from build123d import *

# Parameters (mm, degrees)
BOSS_EXTRUDE1_START = 5
BOSS_EXTRUDE1_DEPTH = 1
SKETCH1_4_W         = 1
SKETCH1_4_H         = 4.3053
BOSS_EXTRUDE2_DEPTH = 5
BOSS_EXTRUDE3_DEPTH = 1.5875


with BuildPart() as part:
    # Sketch1 → Boss-Extrude1 (new body)
    with BuildSketch(Plane(origin=(0, 0, 0), x_dir=(1, 0, 0), z_dir=(0, 1, 0)).offset(BOSS_EXTRUDE1_START)):
        Polygon((13.035, -4), (13.035, 4), (18.035, 4), (18.035, 13.796348116), (3.75, 13.796348116), (3.75, -13.796348116), (18.035, -13.796348116), (18.035, -4), align=None)
    extrude(amount=BOSS_EXTRUDE1_DEPTH)

    # Sketch1<4> → Boss-Extrude2 (add)
    with BuildSketch(Plane(origin=(0, 0, 0), x_dir=(1, 0, 0), z_dir=(0, 1, 0))):
        with Locations((4.25, 0)):
            Rectangle(SKETCH1_4_W, SKETCH1_4_H)
        Polygon((3.75, 3.15265), (3.75, 2.15265), (4.75, 2.15265), (4.75, 12.796348116), (17.035, 12.796348116), (18.035, 12.796348116), (18.035, 13.796348116), (3.75, 13.796348116), align=None)
        Polygon((4.75, -2.15265), (3.75, -2.15265), (3.75, -3.15265), (3.75, -13.796348116), (18.035, -13.796348116), (18.035, -12.796348116), (17.035, -12.796348116), (4.75, -12.796348116), align=None)
    extrude(amount=BOSS_EXTRUDE2_DEPTH)

    # Sketch1<5> → Boss-Extrude3 (add)
    with BuildSketch(Plane(origin=(0, 0, 0), x_dir=(1, 0, 0), z_dir=(0, 1, 0))):
        with BuildLine():
            Line((2.303323685, 2.15265), (3.75, 2.15265))
            Line((3.75, 2.15265), (3.75, 3.15265))
            Line((3.75, 3.15265), (0, 3.15265))
            ThreePointArc((0, 3.15265), (1.255517821, 2.891863936), (2.303323685, 2.15265))
        make_face()
        with BuildLine():
            Line((3.75, -2.15265), (3.75, 2.15265))
            Line((3.75, 2.15265), (2.303323685, 2.15265))
            ThreePointArc((2.303323685, 2.15265), (2.932641765, 1.157071434), (3.15265, 0))
            ThreePointArc((3.15265, 0), (2.932641765, -1.157071434), (2.303323685, -2.15265))
            Line((2.303323685, -2.15265), (3.75, -2.15265))
        make_face()
        with BuildLine():
            Line((3.75, -3.15265), (3.75, -2.15265))
            Line((3.75, -2.15265), (2.303323685, -2.15265))
            ThreePointArc((2.303323685, -2.15265), (1.255517821, -2.891863936), (0, -3.15265))
            Line((0, -3.15265), (3.75, -3.15265))
        make_face()
        with BuildLine():
            ThreePointArc((3.15265, 0), (2.932641765, 1.157071434), (2.303323685, 2.15265))
            Line((2.303323685, 2.15265), (0, 2.15265))
            ThreePointArc((0, 2.15265), (1.522153413, 1.522153413), (2.15265, 0))
            ThreePointArc((2.15265, 0), (1.522153413, -1.522153413), (0, -2.15265))
            Line((0, -2.15265), (2.303323685, -2.15265))
            ThreePointArc((2.303323685, -2.15265), (2.932641765, -1.157071434), (3.15265, 0))
        make_face()
        with BuildLine():
            ThreePointArc((0, -2.15265), (-2.15265, 0), (0, 2.15265))
            Line((0, 2.15265), (0, 3.15265))
            ThreePointArc((0, 3.15265), (-3.15265, 0), (0, -3.15265))
            Line((0, -3.15265), (0, -2.15265))
        make_face()
        with BuildLine():
            Line((0, 2.15265), (2.303323685, 2.15265))
            ThreePointArc((2.303323685, 2.15265), (1.255517821, 2.891863936), (0, 3.15265))
            Line((0, 3.15265), (0, 2.15265))
        make_face()
        with BuildLine():
            ThreePointArc((0, -3.15265), (1.255517821, -2.891863936), (2.303323685, -2.15265))
            Line((2.303323685, -2.15265), (0, -2.15265))
            Line((0, -2.15265), (0, -3.15265))
        make_face()
    extrude(amount=BOSS_EXTRUDE3_DEPTH)


solid = part.part
Can you work these out from the model? Positions are in its coordinate system, mm. A direction names the side the tool comes from. Give positions to 0.01 mm unless a question says otherwise; leave off trailing zeros. Loops run counter-clockwise (first coordinate to the right, second up) from the corner with the lowest first, then second, coordinate; pieces in that order, holes last. Notation, with made-up numbers: (-16, -36.5) - (2, -36.5) arc R23 ccw to (2, -4.5) - close; hole circle Ø11 at (30, -18). An arc over 180 degrees is marked (long way). Answer as a JSON object with one key per item and string values.
Q1. If I drill on L1, parallel to Z at x = 16.5, y = 4.45; L2, parallel to X at y = 3.6, z = -11; L3, parallel to X at y = 5.55, z = 10 (3 decimals), over which ranges is the centre line in solid material (lowest first)?
Geometry says:
{"L1": "-13.8 to -12.8, 12.8 to 13.8", "L2": "3.75 to 4.75", "L3": "3.75 to 18.035"}
Q2. Will these pins go through, and if not, where does the flat tip stop? P1, Ø1.7, axis at x = 2, y = 0.5, coming from the -Z side; P2, Ø10.5, axis at x = 13.5, z = -4.5, coming from the -Y side; P3, Ø1, axis at y = 3, z = -9, coming from the -X side.
Geometry says:
{"P1": "z = -3.15", "P2": "y = 5", "P3": "x = 3.75"}
Q3. Imagine slicing it at A-A on y = 0.45. Write out the boundary of the cut face in (x, z) (3 decimals), plus the area to 3 significant figures.
Geometry says:
{"outline": "(0, -3.153) - (3.75, -3.153) - (3.75, -13.796) - (18.035, -13.796) - (18.035, -12.796) - (4.75, -12.796) - (4.75, 12.796) - (18.035, 12.796) - (18.035, 13.796) - (3.75, 13.796) - (3.75, 3.153) - (0, 3.153) arc R3.153 ccw to start; hole circle Ø4.305 at (0, 0)", "area": "78.9 mm²"}
Q4. If we mould it in two halves opening along Z, with no side actions, what happens to faces 1 (the flat face through (11, 5, 0)), 2 (the flat face through (4, 0, 0)), 3 (the flat face through (11, 3, 13.796)), 4 (the flat face through (11, 2, 12.796))? For each: pulls with the +Z half, pulls with the -Z half, needs draft (parallel to the pull), parting line crosses it, or undercut.
Geometry says:
{"face 1": "undercut", "face 2": "needs draft", "face 3": "pulls with the +Z half", "face 4": "undercut"}
Q5. Imagine slicing it at D-D on x = -1.25. Write out the boundary of the cut face in (y, z), plus the area to 3 significant figures.
Geometry says:
{"outline": "(0, -2.89) - (1.59, -2.89) - (1.59, -1.75) - (0, -1.75) - close; (0, 1.75) - (1.59, 1.75) - (1.59, 2.89) - (0, 2.89) - close", "area": "3.62 mm²"}
Q6. Imagine slicing it at B-B on x = 12. Write out the boundary of the cut face in (y, z).
Geometry says:
{"outline": "(0, -13.8) - (6, -13.8) - (6, 13.8) - (0, 13.8) - (0, 12.8) - (5, 12.8) - (5, -12.8) - (0, -12.8) - close"}
Q7. Which directions (+Z, -Z, +X, -X, +Y, -Y) give clear straight access to the entire face, cutting with the end or side of a thin tool? Please do faces 5 (the flat face through (3, 1.588, 0)), 6 (the flat face through (15.6, 5.5, 4)), 7 (the flat face through (2, 1, 3.153)).
Geometry says:
{"face 5": "+Z, -Z, -X, +Y", "face 6": "+X, +Y, -Y", "face 7": "+Z, -X, +Y, -Y"}
Q8. Imagine slicing it at C-C on y = 5.6. Write out the boundary of the cut face in (x, z) (3 decimals).
Geometry says:
{"outline": "(3.75, -13.796) - (18.035, -13.796) - (18.035, -4) - (13.035, -4) - (13.035, 4) - (18.035, 4) - (18.035, 13.796) - (3.75, 13.796) - close"}
